from build123d import *

# Parameters (mm, degrees)
PAD_DEPTH       = 6
POCKET_DEPTH    = 3
SKETCH002_W     = 18.4
SKETCH002_H     = 20.85
POCKET001_DEPTH = 3
SKETCH003_W     = 8
SKETCH003_H     = 1.65
POCKET002_DEPTH = 3
SKETCH004_W     = 185.077476
SKETCH004_H     = 5.85
PAD001_DEPTH    = 3
SKETCH005_W     = 170.5
SKETCH005_H     = 5.95
PAD002_DEPTH    = 3
SKETCH007_R     = 0.8
POCKET003_DEPTH = 563.341185


with BuildPart() as part:
    # Sketch → Pad (new body)
    with BuildSketch(Plane.XY):
        with BuildLine():
            ThreePointArc((-95, 37.5), (-132.5, 0), (-95, -37.5))
            Line((-95, -37.5), (95, -37.5))
            ThreePointArc((95, -37.5), (132.5, 0), (95, 37.5))
            Line((-95, 37.5), (95, 37.5))
        make_face()
    extrude(amount=PAD_DEPTH)

    # Sketch001 (on Face6 of Pad) → Pocket (cut)
    with BuildSketch(Plane.XY.offset(6)):
        with BuildLine():
            ThreePointArc((-87.3, 6), (-93.3, 0), (-87.3, -6))
            Line((-87.3, -6), (87.3, -6))
            ThreePointArc((87.3, -6), (93.3, 0), (87.3, 6))
            Line((-87.3, 6), (87.3, 6))
        make_face()
    extrude(amount=-POCKET_DEPTH, mode=Mode.SUBTRACT)

    # Sketch002 (on Face5 of Pocket) → Pocket001 (cut)
    with BuildSketch(Plane.XY.offset(6)):
        with Locations((0, -25.425)):
            Rectangle(SKETCH002_W, SKETCH002_H)
    extrude(amount=-POCKET001_DEPTH, mode=Mode.SUBTRACT)

    # Sketch003 (on Face5 of Pocket001) → Pocket002 (cut)
    with BuildSketch(Plane.XY.offset(6)):
        with Locations((0, -36.675)):
            Rectangle(SKETCH003_W, SKETCH003_H)
    extrude(amount=-POCKET002_DEPTH, mode=Mode.SUBTRACT)

    # Sketch004 (on Face5 of Pocket002) → Pad001 (join)
    with BuildSketch(Plane.XY.offset(6)):
        with BuildLine():
            ThreePointArc((-95, 37.5), (-132.5, 0), (-95, -37.5))
            Line((-95, -37.5), (95, -37.5))
            ThreePointArc((95, -37.5), (132.5, 0), (95, 37.5))
            Line((-95, 37.5), (95, 37.5))
        make_face()
        Rectangle(SKETCH004_W, SKETCH004_H, mode=Mode.SUBTRACT)
    extrude(amount=PAD001_DEPTH)

    # Sketch005 (on Face12 of Pad001) → Pad002 (join)
    with BuildSketch(Plane.XY.offset(9)):
        with BuildLine():
            ThreePointArc((-95, 37.5), (-132.5, 0), (-95, -37.5))
            Line((-95, -37.5), (95, -37.5))
            ThreePointArc((95, -37.5), (132.5, 0), (95, 37.5))
            Line((-95, 37.5), (95, 37.5))
        make_face()
        Rectangle(SKETCH005_W, SKETCH005_H, mode=Mode.SUBTRACT)
    extrude(amount=PAD002_DEPTH)

    # Sketch007 (on Face20 of Pad002) → Pocket003 (cut, through all)
    with BuildSketch(Plane.XY.offset(12)):
        with Locations((-90, -8)):
            Circle(SKETCH007_R)
        with Locations((-90, 8)):
            Circle(SKETCH007_R)
        with Locations((-76, 8)):
            Circle(SKETCH007_R)
        with Locations((-76, -8)):
            Circle(SKETCH007_R)
    pocket003 = extrude(amount=-POCKET003_DEPTH, mode=Mode.SUBTRACT)

    # Mirrored: Pocket003 across Sketch007 V_Axis
    add(pocket003.mirror(Plane(origin=(0, 0, 12), x_dir=(0, 0, 1), z_dir=(1, 0, 0))), mode=Mode.SUBTRACT)


solid = part.part
Build history of the part. All positions in model axes, mm. A direction names the side the tool comes from. Round coordinates to 2 decimals unless told otherwise and drop trailing zeros. Loops run counter-clockwise (first coordinate to the right, second up) from the corner with the lowest first, then second, coordinate; pieces in that order, holes last. Notation, with made-up numbers: (-11, -14.5) -> (20, -14.5) arc R17 ccw to (20, 0.5) -> close; hole circle Ø4 at (81, 38.5). An arc over 180 degrees is marked (long way). One line per item, written item: value. Start each with the question number.
Q1. Drop flat-ended pins along their axis: pin 1 Ø3.5 at (y, z) = (-22.5, 4.5) entering from +X; pin 2 Ø3 at (y, z) = (-10.5, 6.5) entering from +X; pin 3 Ø3.5 at (y, z) = (1.5, 8) entering from -X; pin 4 Ø1 at (x, y) = (-90, -8) entering from +Z. Give the stop position or say it passes through.
Q2. Probe line 1 along Y through (x, z) = (90, 8.25) (3 decimals); line 2 along Y through (x, z) = (-76, 9) (3 decimals); line 3 along Y through (x, z) = (74, 5.25). List the from-to ranges inside material, lowest first.
Q3. Cut at A-A on x = -101.5. List the corners of the cut face in (y, z).
Q4. 3-axis set-ups, long thin cutter, end or side, ignore diameter. For faces 5 (the face through (-1, -37.5, 7)), 6 (the face through (89, 0, 9)): which of +Z, -Z, +X, -X, +Y, -Y reach the whole face in a straight line?
Q5. Two-plate mould, pull along X, no slides. Class faces 1 (the face through (-2, 9, 12)), 2 (the face through (-89, 0, 9)), 3 (the face through (-93.3, 0.1, 4.5)), 4 (the face through (132.49, -0.82, 5.92)): released by +X, released by -X, zero draft, split by the parting line, or undercut.
Computed:
1. pin 1: x = 126.24
1. pin 2: x = 131.4
1. pin 3: x = -132.5
1. pin 4: through
2. line 1: -37.5 to -8.8, -7.2 to -2.925, 2.925 to 7.2, 8.8 to 37.5
2. line 2: -37.5 to -8.8, -7.2 to -2.975, 2.975 to 7.2, 8.8 to 37.5
2. line 3: -37.5 to -6, 6 to 37.5
3. outline: (-36.93, 0) -> (36.93, 0) -> (36.93, 12) -> (-36.93, 12) -> close
4. face 5: +Z, -Z, +X, -X, -Y
4. face 6: none
5. face 1: zero draft
5. face 2: undercut
5. face 3: undercut
5. face 4: released by +X
